```python
from build123d import *

# Parameters (mm, degrees)
SHAFTS_R              = 2.9
SHAFT_DEPTH           = 14.6
SHAFTEXTENSIONS_R     = 2.6
SHAFT_EXTENSION_DEPTH = 4
TOOTH_DEPTH           = 18.6
TOOTH_CP_COUNT        = 26
SMALLBORES_R          = 0.8
SMALL_BORE_DEPTH      = 4


with BuildPart() as part:
    # ShaftS → SHAFT (new body)
    with BuildSketch(Plane(origin=(0, 0, 0), x_dir=(1, 0, 0), z_dir=(0, 1, 0))):
        Circle(SHAFTS_R)
    extrude(amount=SHAFT_DEPTH)

    # ShaftExtensionS → SHAFT EXTENSION (add)
    with BuildSketch(Plane(origin=(0, 14.6, 0), x_dir=(1, 0, 0), z_dir=(0, 1, 0))):
        Circle(SHAFTEXTENSIONS_R)
    extrude(amount=SHAFT_EXTENSION_DEPTH)

    # ToothS → TOOTH (add)
    with BuildSketch(Plane(origin=(0, 18.6, 0), x_dir=(1, 0, 0), z_dir=(0, 1, 0))):
        with BuildLine():
            Line((0, 2.9), (-0.262912611, 2.586672952))
            ThreePointArc((-0.262912611, 2.586672952), (0, 2.6), (0.262912611, 2.586672952))
            Line((0.262912611, 2.586672952), (0, 2.9))
        make_face()
    tooth = extrude(amount=-TOOTH_DEPTH)

    # TOOTH CP: TOOTH ×26 about axis
    tooth_cp_axis = Axis((0, 0, 0), (0, 1, 0))
    for i in range(1, TOOTH_CP_COUNT):
        add(tooth.rotate(tooth_cp_axis, i * 360 / TOOTH_CP_COUNT))

    # SmallBoreS → SMALL BORE (cut)
    with BuildSketch(Plane(origin=(0, 18.6, 0), x_dir=(1, 0, 0), z_dir=(0, 1, 0))):
        Circle(SMALLBORES_R)
    extrude(amount=-SMALL_BORE_DEPTH, mode=Mode.SUBTRACT)

    # TeethChamferS → TEETH CHAMFER (revolve, cut)
    with BuildSketch(Plane(origin=(0, 0, 0), x_dir=(0, 0, -1), z_dir=(1, 0, 0))):
        Polygon((2.9, 18.069669914), (2.9, 18.6), (2.369669914, 18.6), align=None)
    revolve(axis=Axis((0, 18.6, 0), (0, -1, 0)), mode=Mode.SUBTRACT)


solid = part.part
```
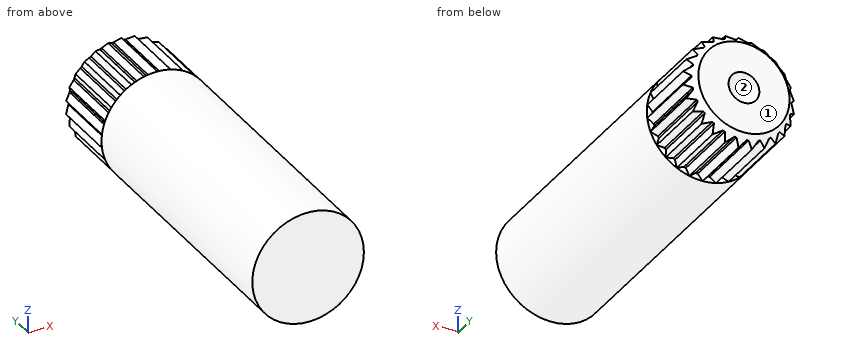
Check sheet for the modelled part. Datum: model origin and axes. Units: mm. Face numbers are marked on the shaded views. A direction names the side the tool comes from. Give positions to 0.01 mm unless a question says otherwise; leave off trailing zeros. Loops run counter-clockwise (first coordinate to the right, second up) from the corner with the lowest first, then second, coordinate; pieces in that order, holes last. Notation, with made-up numbers: (81, 5) - (88, 5) arc R33 ccw to (88, 34) - close; hole circle Ø3 at (86.25, 40). An arc over 180 degrees is marked (long way). One line per question, with ' | ' between items. Start each with the question number.
1. Material ranges on line 1 along X through (y, z) = (15.7, 0); line 2 along Z through (x, y) = (0.7, 2.75); line 3 along X through (y, z) = (18.25, 0.3), recorded low to high. Write a range as [from, to].
2. Set-up check for the marked faces 1 and 2: record each of +Z, -Z, +X, -X, +Y, -Y from which the full face is reachable in a straight line by a thin tool's end or side.
3. Gauge pin test, flat ends, axial feed: pin 1 Ø3 at (y, z) = (2.5, 2) entering from +X; pin 2 Ø1.5 at (y, z) = (3.5, -1) entering from -X; pin 3 Ø1.5 at (x, y) = (-1.5, 16.5) entering from +Z. Record the tip position at first contact, or that the pin passes through.
4. Cross-section at A-A, the plane y = 7.5. Enter the section's corners in (x, z), plus the area to 3 significant figures.
Check result:
1) line 1: x = [-2.6, -0.8], [0.8, 2.6] | line 2: z = [-2.81, 2.81] | line 3: x = [-2.7, -0.74], [0.74, 2.7]
2) face 1: +Z, -Z, +X, -X, +Y | face 2: +Y
3) pin 1: stops at x = 2.86 | pin 2: stops at x = -2.89 | pin 3: stops at z = 2.7
4) outline: circle Ø5.8 at (0, 0) | area: 26.4 mm2
